Model file for the job. Use its own axes, mm. Face numbers are marked on the shaded views. A direction names the side the tool comes from. Give positions to 0.01 mm unless a question says otherwise; leave off trailing zeros. Order: outer loops, then holes, each group sorted by start corner. A loop starts at its lowest first (then second) coordinate and runs counter-clockwise, first axis right, second up. Notation, with made-up numbers: M -15,52.25 L -9,52.25 A25 ccw -9,77.25 Z; hole C 25,11 d4. An arc over 180 degrees is marked long. Return JSON: item names as keys, results as strings. Group by question number.
1. Slice it at C-C on z = 6. List the corners of the cut face in (x, y).
2. Slice it at A-A on y = 0. List the corners of the cut face in (x, z).
3. Wall check: probe 1 along Z at (x, y) = (-3, -2.25); probe 2 along Z at (x, y) = (3, -6.5); probe 3 along Y at (x, z) = (-2.75, 18.5). Give the ranges that are in metal, low to high. Write a range as [from, to].
4. Pin check, flat tips, straight feed: pin 1 (10 mm diameter, centred on y = -4, z = 27.5, fed in from -X); pin 2 (1.5 mm diameter, centred on x = 1.5, z = 26, fed in from -Y); pin 3 (5 mm diameter, centred on x = -3, z = 21, fed in from +Y); pin 4 (10 mm diameter, centred on x = -8.5, z = 34.5, fed in from +Y). Stop position of each tip, or through.
5. 3-axis set-ups, long thin cutter, end or side, ignore diameter. For the marked faces 1 and 2: which of +Z, -Z, +X, -X, +Y, -Y reach the whole face in a straight line?
from build123d import *

# Parameters (mm, degrees)
ESQUISSE1_R        = 13.85
BOSS_EXTRU_1_DEPTH = 27
CHANFREIN1_SIZE    = 5
ESQUISSE2_R        = 1.5
BOSS_EXTRU_2_DEPTH = 13
ESQUISSE3_R        = 4.860209202
BOSS_EXTRU_3_DEPTH = 2


with BuildPart() as part:
    # Esquisse1 → Boss.-Extru.1 (new body)
    with BuildSketch(Plane.XY):
        Circle(ESQUISSE1_R)
    extrude(amount=BOSS_EXTRU_1_DEPTH)

    # Chanfrein1
    chanfrein1_edges = [part.edges().sort_by_distance(p)[0] for p in [
        (-13.85, 0, 27),
    ]]
    chamfer(chanfrein1_edges, length=CHANFREIN1_SIZE)

    # Esquisse2 → Boss.-Extru.2 (add)
    with BuildSketch(Plane.XY.offset(27)):
        with Locations(Location((0, 0, 0), (0, 0, 180))):
            Circle(ESQUISSE2_R)
    extrude(amount=BOSS_EXTRU_2_DEPTH)

    # Esquisse3 → Boss.-Extru.3 (add)
    with BuildSketch(Plane.XY.offset(27)):
        Circle(ESQUISSE3_R)
    extrude(amount=BOSS_EXTRU_3_DEPTH)


solid = part.part
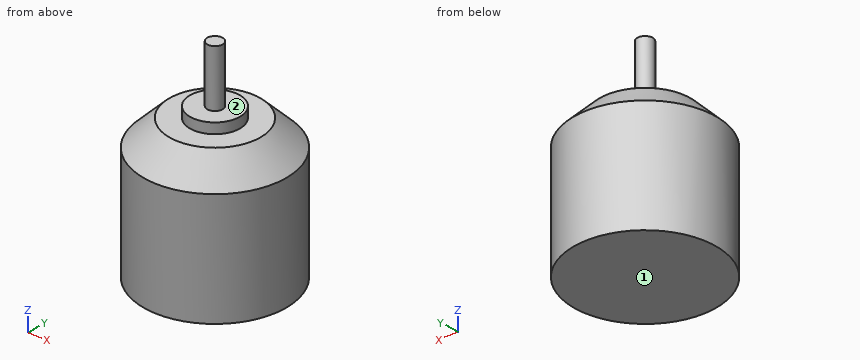
Result:
{
 "1": {"outline": "C 0,0 d27.7"},
 "2": {"outline": "M -13.85,0 L 13.85,0 L 13.85,22 L 8.85,27 L 4.86,27 L 4.86,29 L 1.5,29 L 1.5,40 L -1.5,40 L -1.5,29 L -4.86,29 L -4.86,27 L -8.85,27 L -13.85,22 Z"},
 "3": {"probe 1": "z = [0, 29]", "probe 2": "z = [0, 27]", "probe 3": "y = [-13.57, 13.57]"},
 "4": {"pin 1": "stops at x = -12.91", "pin 2": "stops at y = -10.5", "pin 3": "stops at y = 13.84", "pin 4": "passes through"},
 "5": {"face 1": "-Z, +X, -X, +Y, -Y", "face 2": "+Z"}
}
